```python
from build123d import *

# Parameters (mm, degrees)
F0_W     = 31.5761379898
F0_H     = 78.8946151733
F1_DEPTH = 60
F2_W     = 23.5761379898
F2_H     = 52
F3_DEPTH = 72
F5_DEPTH = 60


with BuildPart() as f1:
    # F0 (on Front) → F1 (new body)
    with BuildSketch(Plane.XZ):
        with Locations((15.7880689949, 39.4473075867)):
            Rectangle(F0_W, F0_H)
    extrude(amount=F1_DEPTH)

    # F2 (on face) → F3 (cut)
    with BuildSketch(Plane.XY.offset(78.8946151733)):
        with Locations((15.7880689949, -30)):
            Rectangle(F2_W, F2_H)
    extrude(amount=-F3_DEPTH, mode=Mode.SUBTRACT)

    # F4 (on face) → F5 (join)
    with BuildSketch(Plane.XZ.offset(60)):
        Polygon((51.5761379898, 78.8946151733), (31.5761379898, 78.8946151733), (31.5761379898, 73.8946151733), (46.5761379898, 73.8946151733), (46.5761379898, 58.8946151733), (51.5761379898, 58.8946151733), align=None)
    extrude(amount=-F5_DEPTH)


solid = f1.part
```
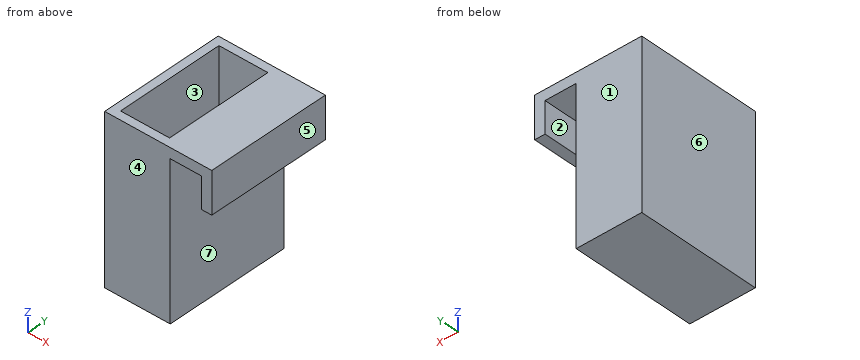
For this review, take the finished solid that the model builds, in its own axes (mm). Face numbers are marked on the shaded views. A direction names the side the tool comes from. Coordinates: 2 decimals unless noted, no trailing zeros. Loops run counter-clockwise (first coordinate to the right, second up) from the corner with the lowest first, then second, coordinate; pieces in that order, holes last.
1. Mouldability with a two-part tool opening along X and no side actions: class the marked faces 4, 5, 6 and 7 as +X half, -X half, draft (parallel to the pull), parting line (faces both ways), or undercut.
2. Add section D-D, the plane y = -34. Give the boundary of the cut face in (x, z).
3. Add section B-B, the plane x = 24.5. Give the boundary of the cut face in (y, z), then the cut area to 3 significant figures.
4. For line 1 (X direction, y = -19, z = 34.5); line 2 (Y direction, x = 24.5, z = 49.5); line 3 (Z direction, x = 7, y = -26.5), list the stretches that pass through material, from the lowest coordinate up.
5. For the marked faces 1, 2 and 3, list the 3-axis set-ups (+Z, -Z, +X, -X, +Y, -Y) from which the entire face can be reached by the end or side of a thin tool; tool diameter is ignored.
6. Insertion check: P1, Ø16.5, axis at x = 41, y = -17, coming from the -Z side; P2, Ø7, axis at x = 17, y = -22.5, coming from the +Z side. Each pin has a flat end and moves straight along its axis. Give the tip position at first contact, or say it passes through.
7. Add section A-A, the plane z = 68. Give the boundary of the cut face in (x, y), then the cut area to 3 significant figures.
8. Add section C-C, the plane z = 31. Give the boundary of the cut face in (x, y).
Result:
1. face 4: draft
1. face 5: +X half
1. face 6: -X half
1. face 7: undercut
2. outline: (0, 0) - (31.58, 0) - (31.58, 73.89) - (46.58, 73.89) - (46.58, 58.89) - (51.58, 58.89) - (51.58, 78.89) - (27.58, 78.89) - (27.58, 6.89) - (4, 6.89) - (4, 78.89) - (0, 78.89) - close
3. outline: (-60, 0) - (0, 0) - (0, 78.89) - (-4, 78.89) - (-4, 6.89) - (-56, 6.89) - (-56, 78.89) - (-60, 78.89) - close
3. area: 990 mm2
4. line 1: x = 0 to 4, 27.58 to 31.58
4. line 2: y = -60 to -56, -4 to 0
4. line 3: z = 0 to 6.89
5. face 1: +Z, -Z, +X, -X, +Y
5. face 2: -Z, +Y, -Y
5. face 3: +Z
6. P1: stops at z = 58.89
6. P2: stops at z = 6.89
7. outline: (0, -60) - (31.58, -60) - (31.58, 0) - (0, 0) - close; (46.58, -60) - (51.58, -60) - (51.58, 0) - (46.58, 0) - close; hole (4, -56) - (27.58, -56) - (27.58, -4) - (4, -4) - close
7. area: 969 mm2
8. outline: (0, -60) - (31.58, -60) - (31.58, 0) - (0, 0) - close; hole (4, -56) - (27.58, -56) - (27.58, -4) - (4, -4) - close
